```python
from build123d import *

# Parameters (mm, degrees)
ESQUISSE1_W           = 8
ESQUISSE1_H           = 10
ESQUISSE1_R           = 2
BOSS_EXTRU_1_DEPTH    = 10
TROU_TARAUD_M31_D     = 2.5
TROU_TARAUD_M31_DEPTH = 5
TROU_TARAUD_M31_TIP   = 0.751075774


with BuildPart() as part:
    # Esquisse1 → Boss.-Extru.1 (new body)
    with BuildSketch(Plane(origin=(0, 0, 0), x_dir=(1, 0, 0), z_dir=(0, 1, 0))):
        Rectangle(ESQUISSE1_W, ESQUISSE1_H)
        with Locations(Location((0, 0, 0), (0, 0, 270))):
            Circle(ESQUISSE1_R, mode=Mode.SUBTRACT)
    extrude(amount=BOSS_EXTRU_1_DEPTH)

    # Trou taraudé M31
    with Locations(Plane.XY.offset(5)):
        with Locations((-2.280208153, 7.049723064), (2.280208153, 7.049723064)):
            Hole(TROU_TARAUD_M31_D / 2, depth=TROU_TARAUD_M31_DEPTH)
            with Locations((0, 0, -(TROU_TARAUD_M31_DEPTH + TROU_TARAUD_M31_TIP / 2))):  # 118° drill point
                Cone(0, TROU_TARAUD_M31_D / 2, TROU_TARAUD_M31_TIP, mode=Mode.SUBTRACT)


solid = part.part
```
Here's how the part is built. I have some questions about the finished solid (model axes, mm). A direction names the side the tool comes from. Coordinates: 2 decimals unless noted, no trailing zeros. Order: outer loops, then holes, each group sorted by start corner. A loop starts at its lowest first (then second) coordinate and runs counter-clockwise, first axis right, second up.
Item 1: If we section it at B-B, the plane y = 3: List the corners of the cut face in (x, z) for me, then the cut area to 3 significant figures.
Response values:
outline: (-4, -5) - (4, -5) - (4, 5) - (-4, 5) - close; hole circle Ø4 at (0, 0)
area: 67.4 mm2
Item 2: If we section it at A-A, the plane x = 0: List the corners of the cut face in (y, z) for me, then the cut area to 3 significant figures.
Response values:
outline: (0, -5) - (10, -5) - (10, -2) - (0, -2) - close; (0, 2) - (10, 2) - (10, 5) - (0, 5) - close
area: 60.0 mm2
Item 3: Which directions (+Z, -Z, +X, -X, +Y, -Y) give clear straight access to the entire face, cutting with the end or side of a thin tool? Please do faces 1 (the face through (-3.47, 7.43, 2.46)), 2 (the face through (4, 5, 0)).
Response values:
face 1: +Z
face 2: +Z, -Z, +X, +Y, -Y
Item 4: If we section it at C-C, the plane z = -1.5: List the corners of the cut face in (x, y) for me.
Response values:
outline: (-4, 0) - (-1.32, 0) - (-1.32, 10) - (-4, 10) - close; (1.32, 0) - (4, 0) - (4, 10) - (1.32, 10) - close
Item 5: Thinking about a two-plate mould opening in Y: for faces 3 (the face through (-2.636, 7.065, -0.537)), 4 (the face through (-2, 0, 1)), 5 (the face through (-4, 5, 0)), which applies, pulls with the +Y half, pulls with the -Y half, needs draft (parallel to the pull), parting line crosses it, or undercut?
Response values:
face 3: undercut
face 4: pulls with the -Y half
face 5: needs draft
Item 6: I need wall thicknesses on probe 1 along Z at (x, y) = (-0.5, 5.5); probe 2 along X at (y, z) = (6.5, -1); probe 3 along Z at (x, y) = (0.25, 4.25). Which ranges of each line are inside material? Lowest first, please.
Response values:
probe 1: z = -5 to -1.94, 1.94 to 5
probe 2: x = -4 to -1.73, 1.73 to 4
probe 3: z = -5 to -1.98, 1.98 to 5
